Geometry check sheet. Reference: the model listing, model coordinates, mm. Face numbers are marked on the shaded views. A direction names the side the tool comes from. Round coordinates to 2 decimals unless told otherwise and drop trailing zeros. Order: outer loops, then holes, each group sorted by start corner. A loop starts at its lowest first (then second) coordinate and runs counter-clockwise, first axis right, second up. Notation, with made-up numbers: (49.5, 27.25) - (106.5, 27.25) arc R21 ccw to (106.5, 63.25) - close; hole circle Ø10 at (46.25, -19.75). An arc over 180 degrees is marked (long way). One line per question, with ' | ' between items. Start each with the question number.
Q1. Sectioned sample at A-A, the plane x = 0. Enter the section's corners in (y, z), then the cut area to 3 significant figures.
Q2. Material ranges on line 1 along Y through (x, z) = (14.5, -9.5); line 2 along Y through (x, z) = (0, -12.25); line 3 along Y through (x, z) = (8.5, -13.75), recorded low to high.
Q3. Sectioned sample at C-C, the plane z = -7.5. Give the number of separate pieces and of enclosed holes in the cut face, then the cut area to 3 significant figures.
Q4. Mould release check, pull along Y, two halves, no side actions. Record for the marked faces 1, 2 and 3: +Y half, -Y half, draft (parallel to the pull), parting line (faces both ways), or undercut.
Q5. Gauge pin test, flat ends, axial feed: P1, Ø5.5, axis at x = 14.5, y = -14.5, coming from the +Z side; P2, Ø1, axis at y = -3, z = -6, coming from the +X side; P3, Ø1.5, axis at x = -1, z = -9.5, coming from the +Y side; P4, Ø11, axis at x = 14.5, y = 14.5, coming from the -Z side. Record the tip position at first contact, or that the pin passes through.
Q6. Tool access check on the marked faces 4, 5 and 6. Record the directions out of +Z, -Z, +X, -X, +Y, -Y that give a thin tool (end or side, any length) a straight path to the whole face; none if there is none.
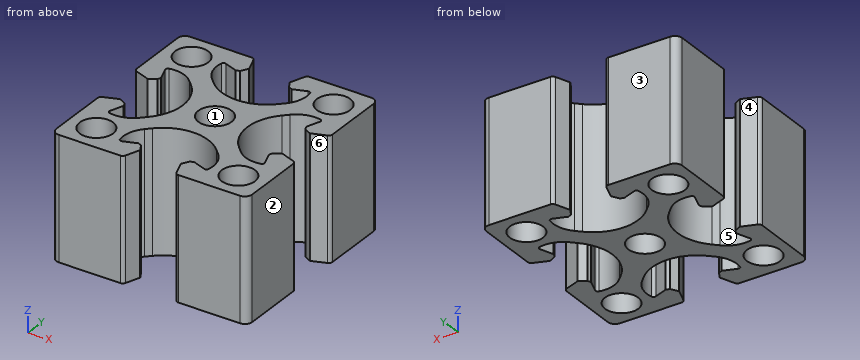
```python
from build123d import *

# Parameters (mm, degrees)
SK_MAIN_EXTRUSION_R  = 3.4
MAIN_EXTRUSION_DEPTH = 25


with BuildPart() as part:
    # Sk Main Extrusion → Main Extrusion (new body)
    with BuildSketch(Plane.XY):
        with BuildLine():
            Line((4.190076845, -16.671180212), (5.222054351, -19.506515107))
            ThreePointArc((5.222054351, -19.506515107), (5.496641489, -19.864364033), (5.926823816, -20))
            Line((5.926823816, -20), (18.5, -20))
            ThreePointArc((18.5, -20), (19.560660172, -19.560660172), (20, -18.5))
            Line((20, -18.5), (20, -5.926823816))
            ThreePointArc((20, -5.926823816), (19.864364033, -5.496641489), (19.506515107, -5.222054351))
            Line((19.506515107, -5.222054351), (16.671180212, -4.190076845))
            ThreePointArc((16.671180212, -4.190076845), (16.563886241, -4.175951325), (16.460675177, -4.208493649))
            Line((16.460675177, -4.208493649), (15.111296024, -4.987558066))
            Line((15.111296024, -4.987558066), (14.845251581, -5.718509166))
            Line((14.845251581, -5.718509166), (15.81984631, -8.396186179))
            ThreePointArc((15.81984631, -8.396186179), (15.786489799, -8.811074612), (15.450654467, -9.056960151))
            ThreePointArc((15.450654467, -9.056960151), (12.665882372, -8.933433013), (10.272684887, -7.504160339))
            Line((10.272684887, -7.504160339), (9.309262274, -6.540737726))
            ThreePointArc((9.309262274, -6.540737726), (6.6, 0), (9.309262274, 6.540737726))
            Line((9.309262274, 6.540737726), (10.272684887, 7.504160339))
            ThreePointArc((10.272684887, 7.504160339), (12.665882372, 8.933433013), (15.450654467, 9.056960151))
            ThreePointArc((15.450654467, 9.056960151), (15.786489799, 8.811074612), (15.81984631, 8.396186179))
            Line((15.81984631, 8.396186179), (14.845251581, 5.718509166))
            Line((14.845251581, 5.718509166), (15.111296024, 4.987558066))
            Line((15.111296024, 4.987558066), (16.460675177, 4.208493649))
            ThreePointArc((16.460675177, 4.208493649), (16.563886241, 4.175951325), (16.671180212, 4.190076845))
            Line((16.671180212, 4.190076845), (19.506515107, 5.222054351))
            ThreePointArc((19.506515107, 5.222054351), (19.864364033, 5.496641489), (20, 5.926823816))
            Line((20, 5.926823816), (20, 18.5))
            ThreePointArc((20, 18.5), (19.560660172, 19.560660172), (18.5, 20))
            Line((18.5, 20), (5.926823816, 20))
            ThreePointArc((5.926823816, 20), (5.496641489, 19.864364033), (5.222054351, 19.506515107))
            Line((5.222054351, 19.506515107), (4.190076845, 16.671180212))
            ThreePointArc((4.190076845, 16.671180212), (4.175951325, 16.563886241), (4.208493649, 16.460675177))
            Line((4.208493649, 16.460675177), (4.987558066, 15.111296024))
            Line((4.987558066, 15.111296024), (5.718509166, 14.845251581))
            Line((5.718509166, 14.845251581), (8.396186179, 15.81984631))
            ThreePointArc((8.396186179, 15.81984631), (8.811074612, 15.786489799), (9.056960151, 15.450654467))
            ThreePointArc((9.056960151, 15.450654467), (8.933433013, 12.665882372), (7.504160339, 10.272684887))
            Line((7.504160339, 10.272684887), (6.540737726, 9.309262274))
            ThreePointArc((6.540737726, 9.309262274), (0, 6.6), (-6.540737726, 9.309262274))
            Line((-6.540737726, 9.309262274), (-7.504160339, 10.272684887))
            ThreePointArc((-7.504160339, 10.272684887), (-8.933433013, 12.665882372), (-9.056960151, 15.450654467))
            ThreePointArc((-9.056960151, 15.450654467), (-8.811074612, 15.786489799), (-8.396186179, 15.81984631))
            Line((-8.396186179, 15.81984631), (-5.718509166, 14.845251581))
            Line((-5.718509166, 14.845251581), (-4.987558066, 15.111296024))
            Line((-4.987558066, 15.111296024), (-4.208493649, 16.460675177))
            ThreePointArc((-4.208493649, 16.460675177), (-4.175951325, 16.563886241), (-4.190076845, 16.671180212))
            Line((-4.190076845, 16.671180212), (-5.222054351, 19.506515107))
            ThreePointArc((-5.222054351, 19.506515107), (-5.496641489, 19.864364033), (-5.926823816, 20))
            Line((-5.926823816, 20), (-18.5, 20))
            ThreePointArc((-18.5, 20), (-19.560660172, 19.560660172), (-20, 18.5))
            Line((-20, 18.5), (-20, 5.926823816))
            ThreePointArc((-20, 5.926823816), (-19.864364033, 5.496641489), (-19.506515107, 5.222054351))
            Line((-19.506515107, 5.222054351), (-16.671180212, 4.190076845))
            ThreePointArc((-16.671180212, 4.190076845), (-16.563886241, 4.175951325), (-16.460675177, 4.208493649))
            Line((-16.460675177, 4.208493649), (-15.111296024, 4.987558066))
            Line((-15.111296024, 4.987558066), (-14.845251581, 5.718509166))
            Line((-14.845251581, 5.718509166), (-15.81984631, 8.396186179))
            ThreePointArc((-15.81984631, 8.396186179), (-15.786489799, 8.811074612), (-15.450654467, 9.056960151))
            ThreePointArc((-15.450654467, 9.056960151), (-12.665882372, 8.933433013), (-10.272684887, 7.504160339))
            Line((-10.272684887, 7.504160339), (-9.309262274, 6.540737726))
            ThreePointArc((-9.309262274, 6.540737726), (-6.6, 0), (-9.309262274, -6.540737726))
            Line((-9.309262274, -6.540737726), (-10.272684887, -7.504160339))
            ThreePointArc((-10.272684887, -7.504160339), (-12.665882372, -8.933433013), (-15.450654467, -9.056960151))
            ThreePointArc((-15.450654467, -9.056960151), (-15.786489799, -8.811074612), (-15.81984631, -8.396186179))
            Line((-15.81984631, -8.396186179), (-14.845251581, -5.718509166))
            Line((-14.845251581, -5.718509166), (-15.111296024, -4.987558066))
            Line((-15.111296024, -4.987558066), (-16.460675177, -4.208493649))
            ThreePointArc((-16.460675177, -4.208493649), (-16.563886241, -4.175951325), (-16.671180212, -4.190076845))
            Line((-16.671180212, -4.190076845), (-19.506515107, -5.222054351))
            ThreePointArc((-19.506515107, -5.222054351), (-19.864364033, -5.496641489), (-20, -5.926823816))
            Line((-20, -5.926823816), (-20, -18.5))
            ThreePointArc((-20, -18.5), (-19.560660172, -19.560660172), (-18.5, -20))
            Line((-18.5, -20), (-5.926823816, -20))
            ThreePointArc((-5.926823816, -20), (-5.496641489, -19.864364033), (-5.222054351, -19.506515107))
            Line((-5.222054351, -19.506515107), (-4.190076845, -16.671180212))
            ThreePointArc((-4.190076845, -16.671180212), (-4.175951325, -16.563886241), (-4.208493649, -16.460675177))
            Line((-4.208493649, -16.460675177), (-4.987558066, -15.111296024))
            Line((-4.987558066, -15.111296024), (-5.718509166, -14.845251581))
            Line((-5.718509166, -14.845251581), (-8.396186179, -15.81984631))
            ThreePointArc((-8.396186179, -15.81984631), (-8.811074612, -15.786489799), (-9.056960151, -15.450654467))
            ThreePointArc((-9.056960151, -15.450654467), (-8.933433013, -12.665882372), (-7.504160339, -10.272684887))
            Line((-7.504160339, -10.272684887), (-6.540737726, -9.309262274))
            ThreePointArc((-6.540737726, -9.309262274), (0, -6.6), (6.540737726, -9.309262274))
            Line((6.540737726, -9.309262274), (7.504160339, -10.272684887))
            ThreePointArc((7.504160339, -10.272684887), (8.933433013, -12.665882372), (9.056960151, -15.450654467))
            ThreePointArc((9.056960151, -15.450654467), (8.811074612, -15.786489799), (8.396186179, -15.81984631))
            Line((8.396186179, -15.81984631), (5.718509166, -14.845251581))
            Line((5.718509166, -14.845251581), (4.987558066, -15.111296024))
            Line((4.987558066, -15.111296024), (4.208493649, -16.460675177))
            ThreePointArc((4.208493649, -16.460675177), (4.175951325, -16.563886241), (4.190076845, -16.671180212))
        make_face()
        with Locations((-14.5, -14.5)):
            Circle(SK_MAIN_EXTRUSION_R, mode=Mode.SUBTRACT)
        with Locations((14.5, -14.5)):
            Circle(SK_MAIN_EXTRUSION_R, mode=Mode.SUBTRACT)
        with Locations((14.5, 14.5)):
            Circle(SK_MAIN_EXTRUSION_R, mode=Mode.SUBTRACT)
        with Locations((-14.5, 14.5)):
            Circle(SK_MAIN_EXTRUSION_R, mode=Mode.SUBTRACT)
        Circle(SK_MAIN_EXTRUSION_R, mode=Mode.SUBTRACT)
    extrude(amount=-MAIN_EXTRUSION_DEPTH)


solid = part.part
```
Determined:
1) outline: (-6.6, -25) - (-3.4, -25) - (-3.4, 0) - (-6.6, 0) - close; (3.4, -25) - (6.6, -25) - (6.6, 0) - (3.4, 0) - close | area: 160 mm2
2) line 1: y = -20 to -17.9, -11.1 to -9.17, 9.17 to 11.1, 17.9 to 20 | line 2: y = -6.6 to -3.4, 3.4 to 6.6 | line 3: y = -20 to -15.85, -11.62 to -5.62, 5.62 to 11.62, 15.85 to 20
3) separate pieces: 1 | enclosed holes: 5 | area: 734 mm2
4) face 1: undercut | face 2: draft | face 3: +Y half
5) P1: passes through | P2: stops at x = 7.29 | P3: stops at y = 6.77 | P4: stops at z = -25
6) face 4: +Z, -Z, -X | face 5: +Z, -Z | face 6: +Z, -Z, +X
